Could you check a few things on this model? Use its own coordinates, in mm. A direction names the side the tool comes from. Give positions to 0.01 mm unless a question says otherwise; leave off trailing zeros. Loops run counter-clockwise (first coordinate to the right, second up) from the corner with the lowest first, then second, coordinate; pieces in that order, holes last. Notation, with made-up numbers: (-5, 61) -> (34, 61) arc R14 cw to (34, 75) -> close; hole circle Ø3 at (-29.75, 17). An arc over 180 degrees is marked (long way). Put each result on its own line as item: value.
```python
from build123d import *

# Parameters (mm, degrees)
SKETCH1_W           = 22
SKETCH1_H           = 28
BOSS_EXTRUDE1_DEPTH = 1
SKETCH2_R           = 1.3
CUT_EXTRUDE8_DEPTH  = 24.286262044
SKETCH3_W           = 5
SKETCH3_H           = 6.4
IC_DEPTH            = 1.2
SKETCH4_R           = 0.5
CUT_EXTRUDE9_DEPTH  = 24.368568634


with BuildPart() as part:
    # Sketch1 → Boss-Extrude1 (new body)
    with BuildSketch(Plane(origin=(0, 0, 0), x_dir=(1, 0, 0), z_dir=(0, 1, 0))):
        with Locations((0, 6.5)):
            Rectangle(SKETCH1_W, SKETCH1_H)
    extrude(amount=BOSS_EXTRUDE1_DEPTH)

    # Sketch2 → Cut-Extrude8 (cut, through all)
    with BuildSketch(Plane(origin=(0, 1, 0), x_dir=(1, 0, 0), z_dir=(0, 1, 0))):
        with Locations(Location((-9, -5.5, 0), (0, 0, 270))):
            Circle(SKETCH2_R)
        with Locations(Location((9, -5.5, 0), (0, 0, 270))):
            Circle(SKETCH2_R)
        with Locations(Location((9, 5.5, 0), (0, 0, 270))):
            Circle(SKETCH2_R)
        with Locations(Location((-9, 5.5, 0), (0, 0, 270))):
            Circle(SKETCH2_R)
    extrude(amount=-CUT_EXTRUDE8_DEPTH, mode=Mode.SUBTRACT)

    # Sketch3 → IC (add)
    with BuildSketch(Plane(origin=(0, 1, 0), x_dir=(1, 0, 0), z_dir=(0, 1, 0))):
        Rectangle(SKETCH3_W, SKETCH3_H)
    extrude(amount=IC_DEPTH)

    # Sketch4 → Cut-Extrude9 (cut, through all)
    with BuildSketch(Plane(origin=(0, 2.2, 0), x_dir=(1, 0, 0), z_dir=(0, 1, 0))):
        with Locations(Location((-8.89, 15.46, 0), (0, 0, 270))):
            Circle(SKETCH4_R)
        with Locations(Location((-6.35, 15.46, 0), (0, 0, 270))):
            Circle(SKETCH4_R)
        with Locations(Location((-3.81, 15.46, 0), (0, 0, 270))):
            Circle(SKETCH4_R)
        with Locations(Location((-1.27, 15.46, 0), (0, 0, 270))):
            Circle(SKETCH4_R)
        with Locations(Location((1.27, 15.46, 0), (0, 0, 270))):
            Circle(SKETCH4_R)
        with Locations(Location((3.81, 15.46, 0), (0, 0, 270))):
            Circle(SKETCH4_R)
        with Locations(Location((6.35, 15.46, 0), (0, 0, 270))):
            Circle(SKETCH4_R)
        with Locations(Location((8.89, 15.46, 0), (0, 0, 270))):
            Circle(SKETCH4_R)
        with Locations(Location((-6.35, 18, 0), (0, 0, 270))):
            Circle(SKETCH4_R)
        with Locations(Location((-3.81, 18, 0), (0, 0, 270))):
            Circle(SKETCH4_R)
        with Locations(Location((-1.27, 18, 0), (0, 0, 270))):
            Circle(SKETCH4_R)
        with Locations(Location((1.27, 18, 0), (0, 0, 270))):
            Circle(SKETCH4_R)
        with Locations(Location((3.81, 18, 0), (0, 0, 270))):
            Circle(SKETCH4_R)
        with Locations(Location((6.35, 18, 0), (0, 0, 270))):
            Circle(SKETCH4_R)
        with Locations(Location((8.89, 18, 0), (0, 0, 270))):
            Circle(SKETCH4_R)
        with Locations(Location((-8.89, 18, 0), (0, 0, 270))):
            Circle(SKETCH4_R)
    extrude(amount=-CUT_EXTRUDE9_DEPTH, mode=Mode.SUBTRACT)


solid = part.part
```
1. If we section it at A-A (z = 5.5): List the corners of the cut face in (x, y) for me, then the cut area to 3 significant figures.
Recorded:
outline: (-11, 0) -> (-10.3, 0) -> (-10.3, 1) -> (-11, 1) -> close; (-7.7, 0) -> (7.7, 0) -> (7.7, 1) -> (-7.7, 1) -> close; (10.3, 0) -> (11, 0) -> (11, 1) -> (10.3, 1) -> close
area: 16.8 mm^2
2. If we section it at D-D (z = -0.5): List the corners of the cut face in (x, y) for me.
Recorded:
outline: (-11, 0) -> (11, 0) -> (11, 1) -> (2.5, 1) -> (2.5, 2.2) -> (-2.5, 2.2) -> (-2.5, 1) -> (-11, 1) -> close
3. If we section it at B-B (x = 3.81): List the corners of the cut face in (y, z) for me, then the cut area to 3 significant figures.
Recorded:
outline: (0, -20.5) -> (1, -20.5) -> (1, -18.5) -> (0, -18.5) -> close; (0, -17.5) -> (1, -17.5) -> (1, -15.96) -> (0, -15.96) -> close; (0, -14.96) -> (1, -14.96) -> (1, 7.5) -> (0, 7.5) -> close
area: 26.0 mm^2
4. I'm going to push flat-ended pins straight in: pin 1 (6.5 mm diameter, centred on x = 5, z = -5.5, fed in from +Y); pin 2 (1.6 mm diameter, centred on x = -9, z = 5.5, fed in from -Y) (1 decimal). Where does each tip first touch, or does it pass through?
Recorded:
pin 1: stops at y = 1
pin 2: passes through
5. If we section it at C-C (y = 0.45): Count the separate pieces of the cut face and the enclosed holes in it, then the cut area to 3 significant figures.
Recorded:
separate pieces: 1
enclosed holes: 20
area: 582 mm^2
6. Thinking about a two-plate mould opening in Z: for faces 4 (the face through (-1.12, 0.507, -17.523)), 5 (the face through (1.42, 0.507, -17.523)), 6 (the face through (0, 2.2, 0)), 7 (the face through (-0.2, 0.5, -20.5)), which applies, pulls with the +Z half, pulls with the -Z half, needs draft (parallel to the pull), parting line crosses it, or undercut?
Recorded:
face 4: undercut
face 5: undercut
face 6: needs draft
face 7: pulls with the -Z half
7. For faces 1 (the face through (0, 0, -7)), 2 (the face through (-2.5, 2, 0)), 3 (the face through (2.5, 2, 0)), which set-ups out of +Z, -Z, +X, -X, +Y, -Y let a thin tool reach every point of the face, with its end or its side?
Recorded:
face 1: +Z, -Z, +X, -X, -Y
face 2: +Z, -Z, -X, +Y
face 3: +Z, -Z, +X, +Y
8. I need wall thicknesses on line 1 (Z direction, x = 3.75, y = 0.75); line 2 (Z direction, x = 10, y = 0.6); line 3 (Y direction, x = -10, z = 0.5). Which ranges of each line are inside material? Lowest first, please.
Recorded:
line 1: z = -20.5 to -18.5, -17.5 to -15.96, -14.96 to 7.5
line 2: z = -20.5 to -6.33, -4.67 to 4.67, 6.33 to 7.5
line 3: y = 0 to 1
